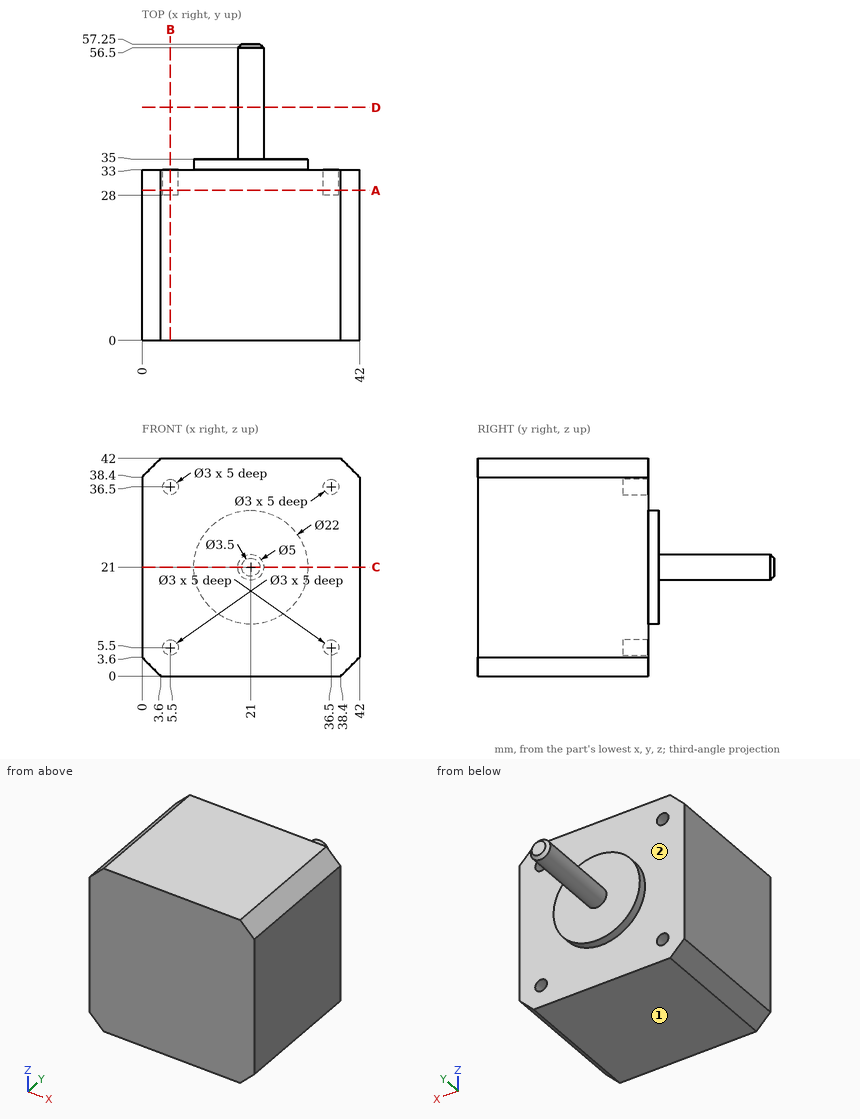
Can you work these out from the drawing? Everything is in mm from the part's minimum corner. A direction names the side the tool comes from. Round coordinates to 2 decimals unless told otherwise and drop trailing zeros. Write each loop counter-clockwise with the first axis right and the second up, starting at its lowest first coordinate (ties: lowest second). Pieces come first, ordered by that corner, then holes.
1. Suppose I cut it at D-D (y = 45). List the corners of the cut face in (x, z) for me, and give its area (3 significant figures).
2. I need wall thicknesses on L1, parallel to X at y = 30, z = 36.5; L2, parallel to X at y = 31, z = 36. Which ranges of each line are inside material? Lowest first, please.
3. Suppose I cut it at A-A (y = 29). List the corners of the cut face in (x, z) for me, and give its area (3 significant figures).
4. Suppose I cut it at C-C (z = 21). List the corners of the cut face in (x, y) for me.
5. Will these pins go through, and if not, where does the flat tip stop? pin 1 Ø4 at (x, z) = (5.5, 5.5) entering from +Y; pin 2 Ø2.5 at (x, z) = (5.5, 36.5) entering from +Y.
6. Suppose I cut it at B-B (x = 5.5). List the corners of the cut face in (y, z) for me.
7. For the marked faces 1 and 2, which set-ups out of +Z, -Z, +X, -X, +Y, -Y let a thin tool reach every point of the face, with its end or its side?
Answer sheet:
1. outline: circle Ø5 at (21, 21)
1. area: 19.6 mm2
2. L1: x = 0 to 4, 7 to 35, 38 to 42
2. L2: x = 0 to 4.09, 6.91 to 35.09, 37.91 to 42
3. outline: (0, 3.6) - (3.6, 0) - (38.4, 0) - (42, 3.6) - (42, 38.4) - (38.4, 42) - (3.6, 42) - (0, 38.4) - close; hole circle Ø3 at (5.5, 5.5); hole circle Ø3 at (5.5, 36.5); hole circle Ø3 at (36.5, 5.5); hole circle Ø3 at (36.5, 36.5)
3. area: 1,710 mm2
4. outline: (0, 0) - (42, 0) - (42, 33) - (32, 33) - (32, 35) - (23.5, 35) - (23.5, 56.5) - (22.75, 57.25) - (19.25, 57.25) - (18.5, 56.5) - (18.5, 35) - (10, 35) - (10, 33) - (0, 33) - close
5. pin 1: stops at y = 33
5. pin 2: stops at y = 28
6. outline: (0, 0) - (33, 0) - (33, 4) - (28, 4) - (28, 7) - (33, 7) - (33, 35) - (28, 35) - (28, 38) - (33, 38) - (33, 42) - (0, 42) - close
7. face 1: -Z, +X, -X, +Y, -Y
7. face 2: +Y
